```python
from build123d import *

# Parameters (mm, degrees)
SKETCH1_W           = 76.2
SKETCH1_H           = 25.4
BOSS_EXTRUDE1_DEPTH = 6.35
SKETCH2_R           = 2.159
CUT_EXTRUDE1_DEPTH  = 41.659838908
SKETCH3_R           = 2.667
CUT_EXTRUDE2_DEPTH  = 41.659838908
SKETCH4_R           = 1.016
CUT_EXTRUDE3_DEPTH  = 7.62
CUT_EXTRUDE4_START  = -7.62
SKETCH5_R           = 1.016
CUT_EXTRUDE4_DEPTH  = 7.62
SKETCH7_R           = 3.302
CUT_EXTRUDE5_DEPTH  = 78.51162816


with BuildPart() as part:
    # Sketch1 → Boss-Extrude1 (new body)
    with BuildSketch(Plane(origin=(0, 0, 0), x_dir=(1, 0, 0), z_dir=(0, 1, 0))):
        Rectangle(SKETCH1_W, SKETCH1_H)
    extrude(amount=BOSS_EXTRUDE1_DEPTH)

    # Sketch2 → Cut-Extrude1 (cut, through all)
    with BuildSketch(Plane(origin=(0, 6.35, 0), x_dir=(1, 0, 0), z_dir=(0, 1, 0))):
        with Locations(Location((-32.074075882, 7.9375, 0), (0, 0, 270))):
            Circle(SKETCH2_R)
        with Locations(Location((-32.074075882, -7.9375, 0), (0, 0, 270))):
            Circle(SKETCH2_R)
        with Locations(Location((31.425924118, 7.9375, 0), (0, 0, 270))):
            Circle(SKETCH2_R)
        with Locations(Location((31.425924118, -7.9375, 0), (0, 0, 270))):
            Circle(SKETCH2_R)
    extrude(amount=-CUT_EXTRUDE1_DEPTH, mode=Mode.SUBTRACT)

    # Sketch3 → Cut-Extrude2 (cut, through all)
    with BuildSketch(Plane(origin=(0, 6.35, 0), x_dir=(1, 0, 0), z_dir=(0, 1, 0))):
        with Locations(Location((-9.525, 7.9375, 0), (0, 0, 270))):
            Circle(SKETCH3_R)
        with Locations(Location((-9.525, -7.9375, 0), (0, 0, 270))):
            Circle(SKETCH3_R)
        with Locations(Location((9.525, 7.9375, 0), (0, 0, 270))):
            Circle(SKETCH3_R)
        with Locations(Location((9.525, -7.9375, 0), (0, 0, 270))):
            Circle(SKETCH3_R)
    extrude(amount=-CUT_EXTRUDE2_DEPTH, mode=Mode.SUBTRACT)

    # Sketch4 → Cut-Extrude3 (cut)
    with BuildSketch(Plane.XY.offset(12.7)):
        with Locations((0, 3.175)):
            Circle(SKETCH4_R)
    extrude(amount=-CUT_EXTRUDE3_DEPTH, mode=Mode.SUBTRACT)

    # Sketch5 → Cut-Extrude4 (cut)
    with BuildSketch(Plane(origin=(0, 0, -12.7), x_dir=(-1, 0, 0), z_dir=(0, 0, -1)).offset(CUT_EXTRUDE4_START)):
        with Locations(Location((0, 3.175, 0), (0, 0, 180))):
            Circle(SKETCH5_R)
    extrude(amount=CUT_EXTRUDE4_DEPTH, mode=Mode.SUBTRACT)

    # Sketch7 → Cut-Extrude5 (cut, through all)
    with BuildSketch(Plane(origin=(38.1, 0, 0), x_dir=(0, 0, -1), z_dir=(1, 0, 0))):
        Circle(SKETCH7_R)
    extrude(amount=-CUT_EXTRUDE5_DEPTH, mode=Mode.SUBTRACT)


solid = part.part
```
For this review, take the finished solid that the model builds, in its own axes (mm). A direction names the side the tool comes from. Give positions to 0.01 mm unless a question says otherwise; leave off trailing zeros. Write each loop counter-clockwise with the first axis right and the second up, starting at its lowest first coordinate (ties: lowest second). Pieces come first, ordered by that corner, then holes.
Item 1: Machinability: for faces 4 (the face through (-12.129, 3.219, -8.516)), 5 (the face through (0, 3, 5.08)), which of the approach directions +Z, -Z, +X, -X, +Y, -Y give a long, thin tool a straight path to every point of the face, cutting with its end or side? Answer none if there is none.
Item 2: Take a section at D-D (x = -15). Give the boundary of the cut face in (y, z).
Item 3: Take a section at B-B (x = 0). Give the boundary of the cut face in (y, z).
Item 4: The part is to be moulded in two halves that separate along Y. For faces 1 (the face through (-11.148, 3.219, 5.821)), 2 (the face through (0, 3, -5.08)), 3 (the face through (0.5, 3.3, -0.1)), say which applies: +Y half, -Y half, draft (parallel to the pull), parting line (faces both ways), or undercut.
Item 5: Take a section at A-A (z = 8.75). Give the boundary of the cut face in (x, y) (3 decimals), and give its area (3 significant figures).
Item 6: Insertion check: P1, Ø1, axis at x = 0, y = 3.5, coming from the +Z side; P2, Ø3.5, axis at x = -32.07, z = 7.94, coming from the +Y side; P3, Ø1.6, axis at x = 0, y = 3.175, coming from the -Z side. Each pin has a flat end and moves straight along its axis. Give the tip position at first contact, or say it passes through.
Item 7: Wall thickness on probe 1 along X at (y, z) = (4.5, -10.25); probe 2 along X at (y, z) = (1, 6.5); probe 3 along X at (y, z) = (0.75, 9.5): over which ranges is each line inside the solid? List them lowest first.
Item 8: Take a section at C-C (z = 0). Give the boundary of the cut face in (x, y), and give its area (3 significant figures).
Established:
1. face 4: +Y, -Y
1. face 5: +Z
2. outline: (0, -12.7) - (6.35, -12.7) - (6.35, 12.7) - (0, 12.7) - (0, 3.3) arc R3.3 cw to (0, -3.3) - close
3. outline: (0, -12.7) - (2.16, -12.7) - (2.16, -5.08) - (4.19, -5.08) - (4.19, -12.7) - (6.35, -12.7) - (6.35, 12.7) - (4.19, 12.7) - (4.19, 5.08) - (2.16, 5.08) - (2.16, 12.7) - (0, 12.7) - (0, 3.3) arc R3.3 cw to (0, -3.3) - close
4. face 1: draft
4. face 2: undercut
4. face 3: -Y half
5. outline: (-38.1, 0) - (-34.074, 0) - (-34.074, 6.35) - (-38.1, 6.35) - close; (-30.074, 0) - (-12.065, 0) - (-12.065, 6.35) - (-30.074, 6.35) - close; (-6.985, 0) - (6.985, 0) - (6.985, 6.35) - (-6.985, 6.35) - close; (12.065, 0) - (29.426, 0) - (29.426, 6.35) - (12.065, 6.35) - close; (33.426, 0) - (38.1, 0) - (38.1, 6.35) - (33.426, 6.35) - close; hole circle Ø2.032 at (0, 3.175)
5. area: 365 mm2
6. P1: stops at z = 5.08
6. P2: passes through
6. P3: stops at z = -5.08
7. probe 1: x = -38.1 to -10.85, -8.2 to 8.2, 10.85 to 38.1
7. probe 2: x = -38.1 to -33.68, -30.46 to -11.77, -7.28 to 7.28, 11.77 to 29.82, 33.04 to 38.1
7. probe 3: x = -38.1 to -33.56, -30.58 to -11.69, -7.36 to 7.36, 11.69 to 29.94, 32.92 to 38.1
8. outline: (-38.1, 3.3) - (38.1, 3.3) - (38.1, 6.35) - (-38.1, 6.35) - close
8. area: 232 mm2
